Work out the finished part from the listing and answer in its coordinate system (mm). A direction names the side the tool comes from. Round coordinates to 2 decimals unless told otherwise and drop trailing zeros. Order: outer loops, then holes, each group sorted by start corner. A loop starts at its lowest first (then second) coordinate and runs counter-clockwise, first axis right, second up. Notation, with made-up numbers: M 38,-10.5 L 46,-10.5 A23 cw 46,14.5 Z; hole C -31,85 d10. An arc over 180 degrees is marked long. Answer as a JSON object with one key per item and string values. Group by question number.
from build123d import *

# Parameters (mm, degrees)
F0_W     = 101.6
F0_H     = 50.8
F1_DEPTH = 6.35
F2_R     = 1.27


with BuildPart() as f1:
    # F0 (on Front) → F1 (new body)
    with BuildSketch(Plane.XZ):
        Rectangle(F0_W, F0_H)
        with BuildLine():
            Line((-25.4, -15.875), (-38.1, -15.875))
            ThreePointArc((-38.1, -15.875), (-41.275, -12.7), (-38.1, -9.525))
            Line((-38.1, -9.525), (-25.4, -9.525))
            ThreePointArc((-25.4, -9.525), (-22.225, -12.7), (-25.4, -15.875))
        make_face(mode=Mode.SUBTRACT)
        with BuildLine():
            Line((25.4, -9.525), (38.1, -9.525))
            ThreePointArc((38.1, -9.525), (41.275, -12.7), (38.1, -15.875))
            Line((38.1, -15.875), (25.4, -15.875))
            ThreePointArc((25.4, -15.875), (22.225, -12.7), (25.4, -9.525))
        make_face(mode=Mode.SUBTRACT)
        with BuildLine():
            Line((-25.4, 9.525), (-38.1, 9.525))
            ThreePointArc((-38.1, 9.525), (-41.275, 12.7), (-38.1, 15.875))
            Line((-38.1, 15.875), (-25.4, 15.875))
            ThreePointArc((-25.4, 15.875), (-22.225, 12.7), (-25.4, 9.525))
        make_face(mode=Mode.SUBTRACT)
        with BuildLine():
            Line((25.4, 15.875), (38.1, 15.875))
            ThreePointArc((38.1, 15.875), (41.275, 12.7), (38.1, 9.525))
            Line((38.1, 9.525), (25.4, 9.525))
            ThreePointArc((25.4, 9.525), (22.225, 12.7), (25.4, 15.875))
        make_face(mode=Mode.SUBTRACT)
    extrude(amount=F1_DEPTH)

    # F2
    f2_edges = [f1.edges().sort_by_distance(p)[0] for p in [
        (0, 0, -25.4),
        (-50.8, 0, 0),
        (50.8, 0, 0),
        (0, 0, 25.4),
        (0, -6.35, 25.4),
        (-50.8, -6.35, 0),
        (50.8, -6.35, 0),
        (0, -6.35, -25.4),
    ]]
    fillet(f2_edges, radius=F2_R)


solid = f1.part
Item 1: A tool of negligible diameter and unlimited length cuts with its end or side. For faces 1 (the cylindrical face through (22.226, -3.131, 12.63)), 2 (the flat face through (50.8, -3, 0)), from which of +Z, -Z, +X, -X, +Y, -Y can it reach the whole face along a straight path? Write none if from no direction.
Item 2: Find section C-C (y = -3.25). Give the vertices of the cut face in (x, z) (3 decimals), and give its area (3 significant figures).
Item 3: Find section B-B (x = 29). Give the vertices of the cut face in (y, z) (3 decimals).
Item 4: This flat-tipped pin is pushed along its axis until it touches: pin 1 (3 mm diameter, centred on x = 26.5, z = -3.5, fed in from +Y). Where does it stop, or does it pass through?
Item 5: Find section A-A (z = -12.7). Give the vertices of the cut face in (x, y) (3 decimals), and give its area (3 significant figures).
Item 6: Consider L1, parallel to Z at x = -35.5, y = -4.25 (3 decimals); L2, parallel to X at y = -2.25, z = -14; L3, parallel to X at y = -0.25, z = 13. Determine where each line is inside the solid, lowest interval first.
Item 7: The mould has two halves that part along Z. Classify faces 3 (the flat face through (-1, -6.35, 0)), 4 (the flat face through (-1, -3, 25.4)), 5 (the cylindrical face through (22.226, -3.131, -12.77)): +Z half, -Z half, draft (parallel to the pull), parting line (faces both ways), or undercut.
Responses:
{
 "1": {"face 1": "+Y, -Y", "face 2": "+Z, -Z, +X, +Y, -Y"},
 "2": {"outline": "M -50.8,-25.4 L 50.8,-25.4 L 50.8,25.4 L -50.8,25.4 Z; hole M -38.1,-15.875 L -25.4,-15.875 A3.175 ccw -25.4,-9.525 L -38.1,-9.525 A3.175 ccw Z; hole M -38.1,9.525 L -25.4,9.525 A3.175 ccw -25.4,15.875 L -38.1,15.875 A3.175 ccw Z; hole M 25.4,-15.875 L 38.1,-15.875 A3.175 ccw 38.1,-9.525 L 25.4,-9.525 A3.175 ccw Z; hole M 25.4,9.525 L 38.1,9.525 A3.175 ccw 38.1,15.875 L 25.4,15.875 A3.175 ccw Z", "area": "4,710 mm^2"},
 "3": {"outline": "M -6.35,-24.13 A1.27 ccw -5.08,-25.4 L -1.27,-25.4 A1.27 ccw 0,-24.13 L 0,-15.875 L -6.35,-15.875 Z; M -6.35,-9.525 L 0,-9.525 L 0,9.525 L -6.35,9.525 Z; M -6.35,15.875 L 0,15.875 L 0,24.13 A1.27 ccw -1.27,25.4 L -5.08,25.4 A1.27 ccw -6.35,24.13 Z"},
 "4": {"pin 1": "stops at y = 0"},
 "5": {"outline": "M -50.8,-5.08 A1.27 ccw -49.53,-6.35 L -41.275,-6.35 L -41.275,0 L -49.53,0 A1.27 ccw -50.8,-1.27 Z; M -22.225,-6.35 L 22.225,-6.35 L 22.225,0 L -22.225,0 Z; M 41.275,-6.35 L 49.53,-6.35 A1.27 ccw 50.8,-5.08 L 50.8,-1.27 A1.27 ccw 49.53,0 L 41.275,0 Z", "area": "402 mm^2"},
 "6": {"L1": "z = -25.4 to -15.875, -9.525 to 9.525, 15.875 to 25.4", "L2": "x = -50.8 to -41, -22.5 to 22.5, 41 to 50.8", "L3": "x = -50.29 to -41.26, -22.24 to 22.24, 41.26 to 50.29"},
 "7": {"face 3": "draft", "face 4": "+Z half", "face 5": "undercut"}
}
